Could you check a few things on this model? Use its own coordinates, in mm. A direction names the side the tool comes from. Round coordinates to 2 decimals unless told otherwise and drop trailing zeros. Put each result on its own line as item: value.
from build123d import *

# Parameters (mm, degrees)
SKETCH1_W                = 1025.461280364
SKETCH1_H                = 19
BOSS_EXTRUDE1_DEPTH      = 250
SKETCH2_R                = 31.474645295
CUT_EXTRUDE1_DEPTH       = 19
SKETCH3_W                = 80
SKETCH3_H                = 19
CUT_EXTRUDE2_DEPTH       = 19
SKETCH4_W                = 80
SKETCH4_H                = 19
CUT_EXTRUDE3_DEPTH       = 19
M5_CLEARANCE_HOLE2_D     = 5.5
M5_CLEARANCE_HOLE2_DEPTH = 19
M5_CLEARANCE_HOLE2_TIP   = 1.652366702


with BuildPart() as part:
    # Sketch1 → Boss-Extrude1 (new body)
    with BuildSketch(Plane.XY):
        with Locations((-1353.189241506, 552.74355083)):
            Rectangle(SKETCH1_W, SKETCH1_H)
    extrude(amount=BOSS_EXTRUDE1_DEPTH)

    # Sketch2 → Cut-Extrude1 (cut)
    with BuildSketch(Plane.XZ.offset(-543.24355083)):
        with Locations((-1759.414463941, 92.370881147)):
            Circle(SKETCH2_R)
    extrude(amount=-CUT_EXTRUDE1_DEPTH, mode=Mode.SUBTRACT)

    # Sketch3 → Cut-Extrude2 (cut)
    with BuildSketch(Plane(origin=(-840.458601324, 0, 0), x_dir=(0, 0, -1), z_dir=(1, 0, 0))):
        with Locations((-120, 552.74355083)):
            Rectangle(SKETCH3_W, SKETCH3_H)
    extrude(amount=-CUT_EXTRUDE2_DEPTH, mode=Mode.SUBTRACT)

    # Sketch4 → Cut-Extrude3 (cut)
    with BuildSketch(Plane.ZY.offset(1865.919881688)):
        with Locations((120, 552.74355083)):
            Rectangle(SKETCH4_W, SKETCH4_H)
    extrude(amount=-CUT_EXTRUDE3_DEPTH, mode=Mode.SUBTRACT)

    # M5 Clearance Hole2
    with Locations(Plane(origin=(-850.780626104, 562.24355083, 20.3), x_dir=(0, 0, 1), z_dir=(0, 1, 0))):
        with Locations((0, 0), (39.7, -178.583190579), (-0.102610802, -347.214178794), (37.25, -508.419165524), (-0.215464176, -729.087144166), (171.700000001, -729.087144166), (171.700000001, -347.214178794), (211.700000001, -171.536855259), (211.700000001, -0.124443922), (211.700000001, -507.967423392), (211.700000001, -827.650747254), (211.700000001, -1005.250659284), (-0.297077663, -1005.250659284), (39.7, -1005.250659284), (38.556814399, 0), (39.7, -823.444523141), (171.625882032, -1006.171227911), (171.900966052, 0.344520361)):
            Hole(M5_CLEARANCE_HOLE2_D / 2, depth=M5_CLEARANCE_HOLE2_DEPTH)
            with Locations((0, 0, -(M5_CLEARANCE_HOLE2_DEPTH + M5_CLEARANCE_HOLE2_TIP / 2))):  # 118° drill point
                Cone(0, M5_CLEARANCE_HOLE2_D / 2, M5_CLEARANCE_HOLE2_TIP, mode=Mode.SUBTRACT)


solid = part.part
(1) Imagine slicing it at A-A, the plane y = 558.25. Give the number of separate pieces and of enclosed holes in the cut face, then the cut area to 3 significant figures.
Values found:
separate pieces: 1
enclosed holes: 19
area: 250,000 mm^2
(2) I'm going to push flat-ended pins straight in: pin 1 (3.5 mm diameter, centred on x = -1022.32, z = 232, fed in from -Y); pin 2 (9.5 mm diameter, centred on y = 555, z = 111.5, fed in from +X). Where does each tip first touch, or does it pass through?
Values found:
pin 1: passes through
pin 2: stops at x = -859.46
(3) For faces 1 (the face through (-1857, 553, 80)), 2 (the face through (-850, 553, 80)), 3 (the face through (-1865.92, 553, 204)), which set-ups out of +Z, -Z, +X, -X, +Y, -Y let a thin tool reach every point of the face, with its end or its side?
Values found:
face 1: -X, +Y, -Y
face 2: +X, +Y, -Y
face 3: +Z, -Z, -X, +Y, -Y
(4) If we mould it in two halves opening along Z, with no side actions, what happens to faces 4 (the face through (-1360, 553, 0)), 5 (the face through (-1360, 543.244, 123)), 6 (the face through (-1360, 553, 250)), 7 (the face through (-1846.92, 553, 119))? For each: pulls with the +Z half, pulls with the -Z half, needs draft (parallel to the pull), parting line crosses it, or undercut.
Values found:
face 4: pulls with the -Z half
face 5: needs draft
face 6: pulls with the +Z half
face 7: undercut
(5) Please list where these lines run through material, in increasing order: probe 1 along Z at (x, y) = (-1361, 549.5); probe 2 along X at (y, z) = (555.75, 60); probe 3 along X at (y, z) = (554, 190). Write a range as from..to.
Values found:
probe 1: z = 0..55.47, 59.63..230.42, 233.58..250
probe 2: x = -1865.92..-1858.78, -1853.28..-1676.98, -1671.48..-1360.45, -1357.95..-1032.11, -1026.61..-853.28, -848.28..-840.46
probe 3: x = -1865.92..-1858.91, -1854.99..-1581.76, -1577.98..-1199.88, -1196.11..-852.08, -848.79..-840.46
